CAD build for the part. Positions are in the model's coordinates, mm. A direction names the side the tool comes from. Give positions to 0.01 mm unless a question says otherwise; leave off trailing zeros. Loops run counter-clockwise (first coordinate to the right, second up) from the corner with the lowest first, then second, coordinate; pieces in that order, holes last.
```python
from build123d import *

# Parameters (mm, degrees)
F1_DEPTH     = 25
F2_R         = 5
F3_T1_DEPTH  = 15
F3_S5_W      = 5
F3_S5_H      = 5
F3_T6_DEPTH  = 5
F3_S11_W     = 5
F3_S11_H     = 5
F3_T12_DEPTH = 5
F4_W         = 36
F4_H         = 1
F4_H_2       = 1.5
F4_H_3       = 2
F5_DEPTH     = 64.1
F7_D         = 6.6
F8_W         = 2
F8_H         = 36
F8_W_2       = 1
F8_W_3       = 1.5
F9_DEPTH     = 69
F11_D        = 6.6


# Not quite as in the source:
# - a fillet or chamfer that OpenCascade refuses, or shapes differently, is made with other operations: its cross-section is extruded or revolved along the edge and cut away or added


with BuildPart() as f1:
    # F0 (on Front) → F1 (new body)
    with BuildSketch(Plane.XZ):
        with BuildLine():
            Line((-200, 0), (0, 0))
            Line((0, 0), (0, 60))
            Line((0, 60), (-137.2273796073, 60))
            Line((-137.2273796073, 60), (-142.2018666706, 54.0716371709))
            ThreePointArc((-142.2018666706, 54.0716371709), (-146.4283628291, 53.7018666706), (-146.7981333294, 57.9283628291))
            Line((-146.7981333294, 57.9283628291), (-140, 66.0300626473))
            Line((-140, 66.0300626473), (-140, 250))
            Line((-140, 250), (-200, 250))
            Line((-200, 250), (-200, 0))
        make_face()
    extrude(amount=F1_DEPTH)

    # F2
    f2_edges = [f1.edges().sort_by_distance(p)[0] for p in [
        (-200, -25, 125),
        (-100, -25, 0),
        (0, -25, 30),
        (-68.61369, -25, 60),
        (-139.714623, -25, 57.035819),
        (-146.428363, -25, 53.701867),
        (-143.399067, -25, 61.979213),
        (-140, -25, 158.015031),
        (-170, -25, 250),
        (-100, 0, 0),
        (-200, -12.5, 0),
        (-200, 0, 125),
        (0, 0, 30),
        (-68.61369, 0, 60),
        (-139.714623, 0, 57.035819),
        (-146.428363, 0, 53.701867),
        (-143.399067, 0, 61.979213),
        (-140, 0, 158.015031),
        (-170, 0, 250),
        (0, -12.5, 0),
        (0, -12.5, 60),
        (-137.22738, -12.5, 60),
        (-140, -12.5, 66.030063),
        (-140, -12.5, 250),
    ]]
    fillet(f2_edges, radius=F2_R)

    # F3: fillet of radius 5 on 1 edges, made by hand

    # F3_s2 → F3_t1 (cut)
    with BuildSketch(Plane.XZ.offset(5)):
        with BuildLine():
            ThreePointArc((-200, 245), (-198.5355339059, 248.5355339059), (-195, 250))
            Line((-195, 250), (-200, 250))
            Line((-200, 250), (-200, 245))
        make_face()
    extrude(amount=F3_T1_DEPTH, mode=Mode.SUBTRACT)


with BuildPart() as f3_tool4:
    # F3_s5 → F3_t6 (new body)
    with BuildSketch(Plane.YZ.offset(-195)):
        with Locations((-2.5, 247.5)):
            Rectangle(F3_S5_W, F3_S5_H)
    extrude(amount=-F3_T6_DEPTH)

    # F3_s7 → F3_t8 (revolve, cut)
    with BuildSketch(Plane(origin=(-195, -5, 245), x_dir=(0, -0.7071067812, -0.7071067812), z_dir=(0, 0.7071067812, -0.7071067812))):
        with BuildLine():
            ThreePointArc((0, -5), (5, 0), (0, 5))
            Line((0, 5), (0, -5))
        make_face()
    revolve(axis=Axis((-195, -5, 245), (-1, 0, 0)), mode=Mode.SUBTRACT)


with BuildPart() as f1_1:
    add(f1.part)

    # F3_t3: cut F3_tool4
    add(f3_tool4.part, mode=Mode.SUBTRACT)


with BuildPart() as f3_tool10:
    # F3_s11 → F3_t12 (new body)
    with BuildSketch(Plane.YZ.offset(-195)):
        with Locations((-22.5, 247.5)):
            Rectangle(F3_S11_W, F3_S11_H)
    extrude(amount=-F3_T12_DEPTH)

    # F3_s13 → F3_t14 (revolve, cut)
    with BuildSketch(Plane(origin=(-195, -20, 245), x_dir=(0, 0.7071067812, -0.7071067812), z_dir=(0, 0.7071067812, 0.7071067812))):
        with BuildLine():
            ThreePointArc((0, -5), (5, 0), (0, 5))
            Line((0, 5), (0, -5))
        make_face()
    revolve(axis=Axis((-195, -20, 245), (-1, 0, 0)), mode=Mode.SUBTRACT)


with BuildPart() as f1_2:
    add(f1_1.part)

    # F3_t9: cut F3_tool10
    add(f3_tool10.part, mode=Mode.SUBTRACT)

    # F4 (on face) → F5 (cut)
    with BuildSketch(Plane(origin=(0, 0, 0), x_dir=(1, 0, 0), z_dir=(0, 0, -1))):
        with Locations((-38, 17)):
            Rectangle(F4_W, F4_H)
        with Locations((-38, 13)):
            Rectangle(F4_W, F4_H_2)
        with Locations((-38, 8.5)):
            Rectangle(F4_W, F4_H_3)
    extrude(amount=-F5_DEPTH, mode=Mode.SUBTRACT)

    # F7 (through all)
    with Locations(Plane(origin=(0, 0, 0), x_dir=(1, 0, 0), z_dir=(0, 0, -1))):
        with Locations((-100, 12.5)):
            Hole(F7_D / 2)

    # F8 (on face) → F9 (cut)
    with BuildSketch(Plane(origin=(-200, 0, 0), x_dir=(0, -1, 0), z_dir=(-1, 0, 0))):
        with Locations((8.5, 212)):
            Rectangle(F8_W, F8_H)
        with Locations((17, 212)):
            Rectangle(F8_W_2, F8_H)
        with Locations((13, 212)):
            Rectangle(F8_W_3, F8_H)
    extrude(amount=-F9_DEPTH, mode=Mode.SUBTRACT)

    # F11 (through all)
    with Locations(Plane(origin=(-200, 0, 0), x_dir=(0, -1, 0), z_dir=(-1, 0, 0))):
        with Locations((12.5, 125)):
            Hole(F11_D / 2)


solid = f1_2.part
```
1. Saw through at A-A, the plane x = -100. List the corners of the cut face in (y, z).
Responses:
outline: (-25, 5) arc R5 ccw to (-20, 0) - (-15.8, 0) - (-15.8, 60) - (-20, 60) arc R5 ccw to (-25, 55) - close; (-9.2, 0) - (-5, 0) arc R5 ccw to (0, 5) - (0, 55) arc R5 ccw to (-5, 60) - (-9.2, 60) - close
2. Saw through at C-C, the plane x = -26.5. List the corners of the cut face in (y, z), and give its area (3 significant figures).
Responses:
outline: (-25, 5) arc R5 ccw to (-20, 0) - (-17.5, 0) - (-17.5, 60) - (-20, 60) arc R5 ccw to (-25, 55) - close; (-16.5, 0) - (-13.75, 0) - (-13.75, 60) - (-16.5, 60) - close; (-12.25, 0) - (-9.5, 0) - (-9.5, 60) - (-12.25, 60) - close; (-7.5, 0) - (-5, 0) arc R5 ccw to (0, 5) - (0, 55) arc R5 ccw to (-5, 60) - (-7.5, 60) - close
area: 1,210 mm2
3. Pull direction X, two halves, no side cores. Call faces 4 (the face through (-200, -9, 127)), 5 (the face through (-38, -17.5, 30)), 6 (the face through (-170, -16.5, 212)): released by +X, released by -X, zero draft, split by the parting line, or undercut.
Responses:
face 4: released by -X
face 5: undercut
face 6: zero draft
4. Saw through at B-B, the plane z = 215.5. List the corners of the cut face in (x, y).
Responses:
outline: (-200, -20) arc R5 ccw to (-195, -25) - (-145, -25) arc R5 ccw to (-140, -20) - (-140, -17.5) - (-200, -17.5) - close; (-200, -16.5) - (-140, -16.5) - (-140, -13.75) - (-200, -13.75) - close; (-200, -12.25) - (-140, -12.25) - (-140, -9.5) - (-200, -9.5) - close; (-200, -7.5) - (-140, -7.5) - (-140, -5) arc R5 ccw to (-145, 0) - (-195, 0) arc R5 ccw to (-200, -5) - close
5. Saw through at D-D, the plane z = 125. List the corners of the cut face in (x, y), and give its area (3 significant figures).
Responses:
outline: (-200, -20) arc R5 ccw to (-195, -25) - (-145, -25) arc R5 ccw to (-140, -20) - (-140, -15.8) - (-200, -15.8) - close; (-200, -9.2) - (-140, -9.2) - (-140, -5) arc R5 ccw to (-145, 0) - (-195, 0) arc R5 ccw to (-200, -5) - close
area: 1,080 mm2
6. Drop flat-ended pins along their axis: pin 1 (8 mm diameter, centred on x = -69.5, y = -11.5, fed in from +Z); pin 2 (1 mm diameter, centred on y = -20, z = 104.5, fed in from +X). Give the stop position or say it passes through.
Responses:
pin 1: stops at z = 60
pin 2: stops at x = -140
7. Probe line 1 along X through (y, z) = (-12.5, 35.5); line 2 along Z through (x, y) = (-178.5, -12.5); line 3 along Y through (x, z) = (-100, 28). List the from-to ranges inside material, lowest first.
Responses:
line 1: x = -200 to -103.3, -96.7 to -56, -20 to 0
line 2: z = 0 to 121.7, 128.3 to 194, 230 to 250
line 3: y = -25 to -15.8, -9.2 to 0
8. Tool access for faces 1 (the face through (-38, -9.5, 30)), 2 (the face through (-139.396, -23.496, 55.197)), 3 (the face through (-69, -12, 60)): list every direction of +Z, -Z, +X, -X, +Y, -Y with a clear straight run to the whole face (end or side of a thin tool).
Responses:
face 1: +Z, -Z
face 2: -Y
face 3: +Z, +X, +Y, -Y
